Can you work these out from the model? Positions are in its coordinate system, mm. A direction names the side the tool comes from. Round coordinates to 2 decimals unless told otherwise and drop trailing zeros. Loops run counter-clockwise (first coordinate to the right, second up) from the corner with the lowest first, then second, coordinate; pieces in that order, holes last.
(1) Will these pins go through, and if not, where does the flat tip stop? pin 1 Ø12 at (x, y) = (30.5, 11.5) entering from +Z; pin 2 Ø4.5 at (y, z) = (22.5, 0) entering from +X; pin 3 Ø4 at (y, z) = (20, -0.5) entering from -X; pin 4 Ø3 at (x, z) = (11.5, -2) entering from +Y.
(2) Thinking about a two-plate mould opening in X: for faces 6 (the face through (21, 21.5, -7.3)), 7 (the face through (21, 4.5, 2)), 8 (the face through (8.4, 2.3, 0.1)), which applies, released by +X, released by -X, zero draft, split by the parting line, or undercut?
(3) Which directions (+Z, -Z, +X, -X, +Y, -Y) give clear straight access to the entire face, cutting with the end or side of a thin tool? Please do faces 1 (the face through (2.3, 8.4, -0.1)), 2 (the face through (13, 2, 2.6)), 3 (the face through (4.5, 21, 2)), 4 (the face through (38, 2, 0)), 5 (the face through (19, 0, 0)).
(4) I want a section at B-B on z = 1. Write out the boundary of the cut face in (x, y).
(5) I want a section at A-A on x = 3.5. Write out the boundary of the cut face in (y, z), plus the area to 3 significant figures.
(6) I want a section at C-C on y = 13.5. Write out the boundary of the cut face in (x, z).
(7) I want a section at D-D on x = 25.5. Write out the boundary of the cut face in (y, z).
(8) If I drill on line 1 along X through (y, z) = (4, 0.25); line 2 along Z through (x, y) = (15, 22); line 3 along Y through (x, z) = (29, 8), over which ranges is the centre line in solid material (lowest first)?
from build123d import *

# Parameters (mm, degrees)
BOSS_EXTRUDE1_DEPTH = 8.75
BOSS_EXTRUDE2_DEPTH = 3
CUT_EXTRUDE1_DEPTH  = 4.5
CUT_EXTRUDE2_DEPTH  = 4.5


with BuildPart() as part:
    # Sketch1 → Boss-Extrude1 (new, symmetric)
    with BuildSketch(Plane.XY):
        Polygon((0, 0), (0, 38), (4.5, 38), (4.5, 4.5), (38, 4.5), (38, 0), align=None)
    extrude(amount=BOSS_EXTRUDE1_DEPTH, both=True)

    # Sketch2 → Boss-Extrude2 (add)
    with BuildSketch(Plane(origin=(0, 0, -8.75), x_dir=(-1, 0, 0), z_dir=(0, 0, -1))):
        Polygon((-4.5, 38), (-38, 4.5), (-38, 0), (0, 0), (0, 38), align=None)
    extrude(amount=-BOSS_EXTRUDE2_DEPTH)

    # Sketch3 → Cut-Extrude1 (cut)
    with BuildSketch(Plane(origin=(0, 4.5, 0), x_dir=(1, 0, 0), z_dir=(0, 1, 0))):
        with BuildLine():
            Line((30, -2.6), (26, -2.6))
            ThreePointArc((26, -2.6), (23.4, 0), (26, 2.6))
            Line((26, 2.6), (30, 2.6))
            ThreePointArc((30, 2.6), (32.6, 0), (30, -2.6))
        make_face()
        with BuildLine():
            Line((11, 2.6), (15, 2.6))
            ThreePointArc((15, 2.6), (17.6, 0), (15, -2.6))
            Line((15, -2.6), (11, -2.6))
            ThreePointArc((11, -2.6), (8.4, 0), (11, 2.6))
        make_face()
    extrude(amount=-CUT_EXTRUDE1_DEPTH, mode=Mode.SUBTRACT)

    # Sketch4 → Cut-Extrude2 (cut)
    with BuildSketch(Plane(origin=(4.5, 0, 0), x_dir=(0, 0, -1), z_dir=(1, 0, 0))):
        with BuildLine():
            Line((2.6, 30), (2.6, 26))
            ThreePointArc((2.6, 26), (0, 23.4), (-2.6, 26))
            Line((-2.6, 26), (-2.6, 30))
            ThreePointArc((-2.6, 30), (0, 32.6), (2.6, 30))
        make_face()
        with BuildLine():
            Line((2.6, 15), (2.6, 11))
            ThreePointArc((2.6, 11), (0, 8.4), (-2.6, 11))
            Line((-2.6, 11), (-2.6, 15))
            ThreePointArc((-2.6, 15), (0, 17.6), (2.6, 15))
        make_face()
    extrude(amount=-CUT_EXTRUDE2_DEPTH, mode=Mode.SUBTRACT)


solid = part.part
Filled sheet:
1. pin 1: stops at z = -5.75
1. pin 2: stops at x = 4.5
1. pin 3: stops at x = 0
1. pin 4: stops at y = 4.5
2. face 6: released by +X
2. face 7: zero draft
2. face 8: undercut
3. face 1: +X, -X
3. face 2: +Y, -Y
3. face 3: +Z, +X, +Y
3. face 4: +Z, -Z, +X, +Y, -Y
3. face 5: +Z, -Z, +X, -X, -Y
4. outline: (0, 0) - (8.6, 0) - (8.6, 4.5) - (4.5, 4.5) - (4.5, 8.6) - (0, 8.6) - close; (0, 17.4) - (4.5, 17.4) - (4.5, 23.6) - (0, 23.6) - close; (0, 32.4) - (4.5, 32.4) - (4.5, 38) - (0, 38) - close; (17.4, 0) - (23.6, 0) - (23.6, 4.5) - (17.4, 4.5) - close; (32.4, 0) - (38, 0) - (38, 4.5) - (32.4, 4.5) - close
5. outline: (0, -8.75) - (38, -8.75) - (38, 8.75) - (0, 8.75) - close; hole (11, -2.6) - (15, -2.6) arc R2.6 ccw to (15, 2.6) - (11, 2.6) arc R2.6 ccw to start; hole (26, -2.6) - (30, -2.6) arc R2.6 ccw to (30, 2.6) - (26, 2.6) arc R2.6 ccw to start
5. area: 581 mm2
6. outline: (0, -8.75) - (29, -8.75) - (29, -5.75) - (4.5, -5.75) - (4.5, -2.6) - (0, -2.6) - close; (0, 2.6) - (4.5, 2.6) - (4.5, 8.75) - (0, 8.75) - close
7. outline: (0, -8.75) - (17, -8.75) - (17, -5.75) - (4.5, -5.75) - (4.5, -2.55) - (0, -2.55) - close; (0, 2.55) - (4.5, 2.55) - (4.5, 8.75) - (0, 8.75) - close
8. line 1: x = 0 to 8.41, 17.59 to 23.41, 32.59 to 38
8. line 2: z = -8.75 to -5.75
8. line 3: y = 0 to 4.5
